```python
from build123d import *

# Parameters (mm, degrees)
ESQUISSE1_W      = 12
ESQUISSE1_H      = 40
EXTRUSION1_DEPTH = 17
EXTRUSION2_DEPTH = 12
ESQUISSE3_W      = 6
ESQUISSE3_H      = 3
EXTRUSION3_DEPTH = 25.083189158
ESQUISSE4_W      = 3
ESQUISSE4_H      = 40
EXTRUSION4_DEPTH = 4


with BuildPart() as part:
    # Esquisse1 → Extrusion1 (new body)
    with BuildSketch(Plane.XY):
        Rectangle(ESQUISSE1_W, ESQUISSE1_H)
    extrude(amount=EXTRUSION1_DEPTH)

    # Esquisse2 → Extrusion2 (cut)
    with BuildSketch(Plane.XY.offset(17)):
        with BuildLine():
            Line((-3, 14.5), (-3, -14.5))
            ThreePointArc((-3, -14.5), (0, -17.5), (3, -14.5))
            Line((3, -14.5), (3, 14.5))
            ThreePointArc((3, 14.5), (0, 17.5), (-3, 14.5))
        make_face()
    extrude(amount=-EXTRUSION2_DEPTH, mode=Mode.SUBTRACT)

    # Esquisse3 → Extrusion3 (cut, through all)
    with BuildSketch(Plane.XY.offset(5)):
        Rectangle(ESQUISSE3_W, ESQUISSE3_H)
    extrude(amount=-EXTRUSION3_DEPTH, mode=Mode.SUBTRACT)

    # Esquisse4 → Extrusion4 (add)
    with BuildSketch(Plane.XY.offset(17)):
        with Locations((4.5, 0)):
            Rectangle(ESQUISSE4_W, ESQUISSE4_H)
        with Locations((-4.5, 0)):
            Rectangle(ESQUISSE4_W, ESQUISSE4_H)
    extrude(amount=EXTRUSION4_DEPTH)


solid = part.part
```
Read the model definition and answer for the solid it produces. Units are mm, in the model's axes. A direction names the side the tool comes from. Coordinates: 2 decimals unless noted, no trailing zeros. Order: outer loops, then holes, each group sorted by start corner. A loop starts at its lowest first (then second) coordinate and runs counter-clockwise, first axis right, second up. Notation, with made-up numbers: (-30.5, 36.25) - (15.5, 36.25) arc R29 ccw to (15.5, 63.25) - close; hole circle Ø9 at (80, 65.5). An arc over 180 degrees is marked (long way). Answer as a JSON object with one key per item and string values. Group by question number.
Item 1: Section B-B (z = 8.75) is taken. Give the vertices of the cut face in (x, y), plus the area to 3 significant figures.
Item 2: Consider probe 1 along X at (y, z) = (7, 14.25); probe 2 along Y at (x, z) = (-2.75, 2.25); probe 3 along Z at (x, y) = (-0.5, 3). Determine where each line is inside the solid, lowest interval first. Write a range as from..to.
Item 3: Section A-A (x = 0) is taken. Give the vertices of the cut face in (y, z).
Item 4: The mould has two halves that part along Y. Classify faces 1 (the face through (-6, 0, 10)), 2 (the face through (0, -1.5, 3)), 3 (the face through (0, -20, 10)): +Y half, -Y half, draft (parallel to the pull), parting line (faces both ways), or undercut.
Item 5: A tool of negligible diameter and unlimited length cuts with its end or side. For faces 4 (the face through (0, 1.5, 3)), 5 (the face through (-0.1, -17.5, 11.1)), 6 (the face through (0, 19, 17)), from which of +Z, -Z, +X, -X, +Y, -Y can it reach the whole face along a straight path? Write none if from no direction.
Item 6: Flat-ended cylindrical pins translate along their axes: P1, Ø1.5, axis at x = 2, y = -16, coming from the +Z side; P2, Ø1.6, axis at x = 0.5, y = 16.5, coming from the +Z side. Find the tip coordinate at first contact, or state that the pin passes through.
Item 7: Section D-D (x = -2.25) is taken. Give the vertices of the cut face in (y, z).
Item 8: Section C-C (y = -3) is taken. Give the vertices of the cut face in (x, z), plus the area to 3 significant figures.
Results are:
{
 "1": {"outline": "(-6, -20) - (6, -20) - (6, 20) - (-6, 20) - close; hole (-3, -14.5) arc R3 ccw to (3, -14.5) - (3, 14.5) arc R3 ccw to (-3, 14.5) - close", "area": "278 mm^2"},
 "2": {"probe 1": "x = -6..-3, 3..6", "probe 2": "y = -20..-1.5, 1.5..20", "probe 3": "z = 0..5"},
 "3": {"outline": "(-20, 0) - (-1.5, 0) - (-1.5, 5) - (-17.5, 5) - (-17.5, 17) - (-20, 17) - close; (1.5, 0) - (20, 0) - (20, 17) - (17.5, 17) - (17.5, 5) - (1.5, 5) - close"},
 "4": {"face 1": "draft", "face 2": "undercut", "face 3": "-Y half"},
 "5": {"face 4": "+Z, -Z", "face 5": "+Z", "face 6": "+Z, +Y, -Y"},
 "6": {"P1": "stops at z = 17", "P2": "stops at z = 5"},
 "7": {"outline": "(-20, 0) - (-1.5, 0) - (-1.5, 5) - (-16.48, 5) - (-16.48, 17) - (-20, 17) - close; (1.5, 0) - (20, 0) - (20, 17) - (16.48, 17) - (16.48, 5) - (1.5, 5) - close"},
 "8": {"outline": "(-6, 0) - (6, 0) - (6, 21) - (3, 21) - (3, 5) - (-3, 5) - (-3, 21) - (-6, 21) - close", "area": "156 mm^2"}
}
